Could you check a few things on this model? Use its own coordinates, in mm. Face numbers are marked on the shaded views. A direction names the side the tool comes from. Round coordinates to 2 decimals unless told otherwise and drop trailing zeros. Write each loop counter-clockwise with the first axis right and the second up, starting at its lowest first coordinate (ties: lowest second). Pieces come first, ordered by that corner, then holes. Notation, with made-up numbers: (15.5, 4.25) - (39.5, 4.25) arc R6 ccw to (39.5, 13.25) - close; hole circle Ø4 at (43.5, -24). An arc over 180 degrees is marked (long way). Write each question's results on one line, items separated by ' | '. Start each with the question number.
(1) On a 3-axis mill with a long thin cutter (end or side, diameter ignored), from which of +Z, -Z, +X, -X, +Y, -Y can I reach the whole of each face in a straight line? I mean the marked faces 4 and 5. Say none if no direction works.
(2) Thinking about a two-plate mould opening in Z: for the marked faces 1, 2 and 3, which applies, +Z half, -Z half, draft (parallel to the pull), parting line (faces both ways), or undercut?
(3) Imagine slicing it at C-C on z = -16.5. Write out the boundary of the cut face in (x, y) (3 decimals).
(4) Imagine slicing it at B-B on x = -0.5. Write out the boundary of the cut face in (y, z).
(5) Please list where these lines run through material, in increasing order: line 1 (Z direction, x = -10.5, y = 16); line 2 (X direction, y = -20, z = 6); line 3 (Y direction, x = -5.5, z = -30.5). Write a range as [from, to].
(6) For P1, Ø10, axis at x = -28.5, z = -3, coming from the +Y side, with a flat end and sliding along its axis, tell me the tip position at first contact or that it passes through.
(7) Imagine slicing it at A-A on y = -15.5. Write out the boundary of the cut face in (x, z), then the cut area to 3 significant figures.
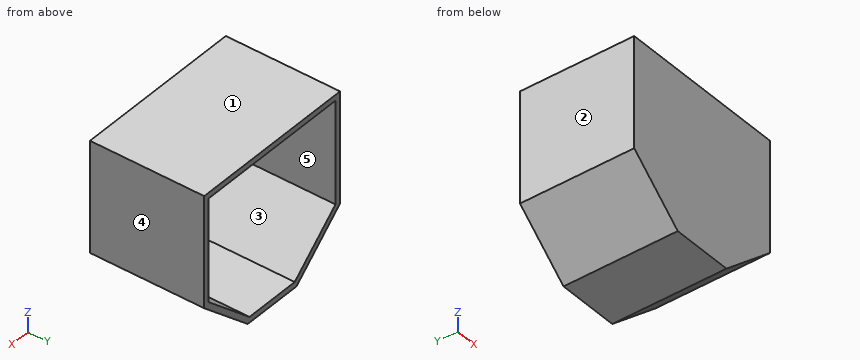
```python
from build123d import *

# Parameters (mm, degrees)
BOSS_EXTRUDE1_DEPTH = 25.4
SHELL1_T            = -2.54


with BuildPart() as part:
    # Sketch2 → Boss-Extrude1 (new, symmetric)
    # profile 1 of 2: a face of its own
    with BuildSketch(Plane(origin=(0, 0, 0), x_dir=(1, 0, 0), z_dir=(0, 1, 0))):
        Polygon((13.665706279, 35.56), (38.1, 13.840627803), (38.1, -35.56), (-38.1, -35.56), (-38.1, 13.840627803), (-13.665706279, 35.56), align=None)
        Polygon((12.7, 33.02), (35.56, 12.7), (35.56, -33.02), (-35.56, -33.02), (-35.56, 12.7), (-12.7, 33.02), align=None, mode=Mode.SUBTRACT)
    # profile 2 of 2: a face of its own
    with BuildSketch(Plane(origin=(0, 0, 0), x_dir=(1, 0, 0), z_dir=(0, 1, 0))):
        Polygon((35.56, 12.7), (35.56, -33.02), (-35.56, -33.02), (-35.56, 12.7), (-12.7, 33.02), (12.7, 33.02), align=None)
    extrude(amount=BOSS_EXTRUDE1_DEPTH, both=True)

    # Shell1
    shell1_openings = [part.faces().sort_by_distance(p)[0] for p in [
        (0, 25.4, 3.07436115),
    ]]
    offset(amount=SHELL1_T, openings=shell1_openings, kind=Kind.INTERSECTION)


solid = part.part
```
Response:
1) face 4: +Z, -Z, +X, +Y, -Y | face 5: +Y
2) face 1: +Z half | face 2: draft | face 3: undercut
3) outline: (-35.108, -25.4) - (35.108, -25.4) - (35.108, 25.4) - (31.285, 25.4) - (31.285, -22.86) - (-31.285, -22.86) - (-31.285, 25.4) - (-35.108, 25.4) - close
4) outline: (-25.4, -35.56) - (25.4, -35.56) - (25.4, -33.02) - (-22.86, -33.02) - (-22.86, 33.02) - (25.4, 33.02) - (25.4, 35.56) - (-25.4, 35.56) - close
5) line 1: [-35.56, -33.02], [33.02, 35.56] | line 2: [-38.1, -35.56], [35.56, 38.1] | line 3: [-25.4, -22.86]
6) P1: y = -22.86
7) outline: (-38.1, -13.84) - (-13.67, -35.56) - (13.67, -35.56) - (38.1, -13.84) - (38.1, 35.56) - (-38.1, 35.56) - close; hole (-35.56, -12.7) - (-12.7, -33.02) - (12.7, -33.02) - (35.56, -12.7) - (35.56, 33.02) - (-35.56, 33.02) - close | area: 656 mm²
